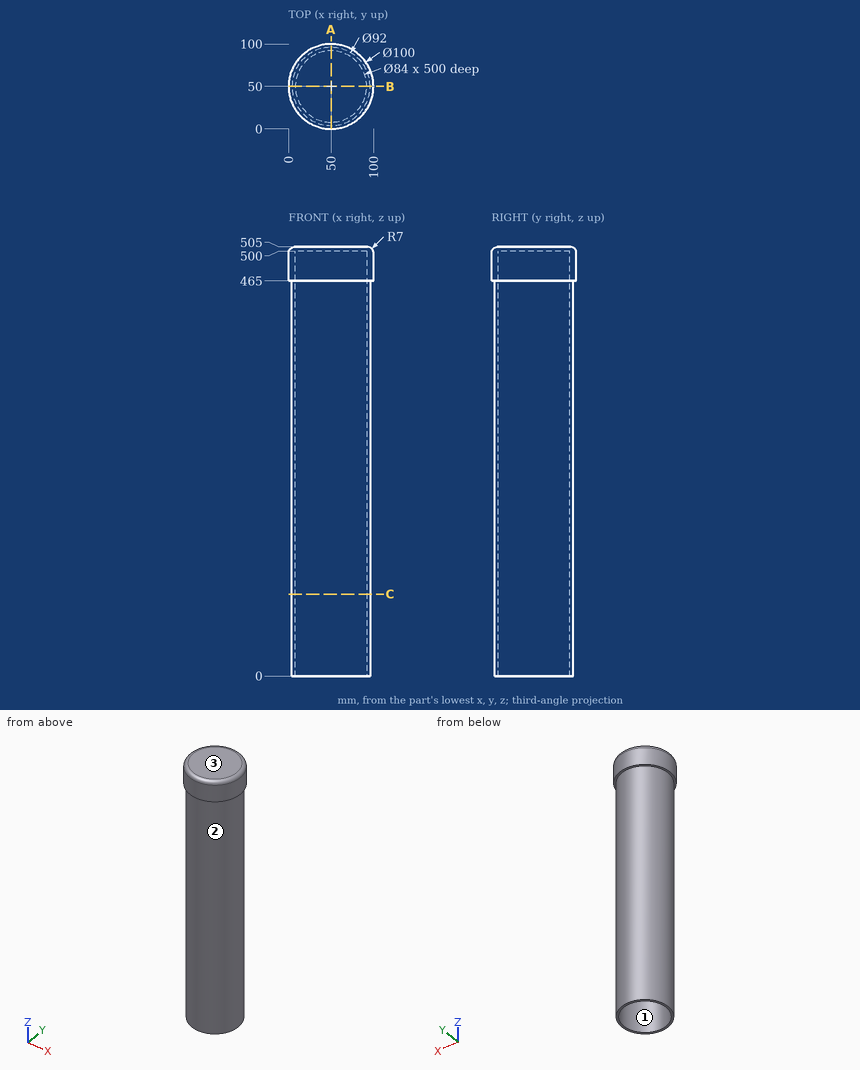
Design review of the part shown in the three views and the two pictorial views. Dimensions are in mm from the part's minimum x, y and z. Round coordinates to 2 decimals unless told otherwise and drop trailing zeros. Loops run counter-clockwise (first coordinate to the right, second up) from the corner with the lowest first, then second, coordinate; pieces in that order, holes last. Notation, with made-up numbers: (32.5, -26.75) - (37.5, -26.75) arc R27 cw to (37.5, -6.75) - close; hole circle Ø7 at (35.5, -34.5). An arc over 180 degrees is marked (long way). Write each question's results on one line, items separated by ' | '. Start each with the question number.
Q1. Take a section at C-C on z = 96.5. Give the boundary of the cut face in (x, y).
Q2. Wall thickness on line 1 along Y through (x, z) = (50, 174); line 2 along Y through (x, z) = (51, 470); line 3 along X through (y, z) = (26, 277): over which ranges is each line inside the solid? List them lowest first. Write a range as [from, to].
Q3. Take a section at A-A on x = 50. Give the boundary of the cut face in (y, z).
Q4. Draft analysis for pull direction Y (two halves, no side actions). For the marked faces 1, 2 and 3, state which applies: pulls with the +Y half, pulls with the -Y half, needs draft (parallel to the pull), parting line crosses it, or undercut.
Q5. Insertion check: P1, Ø25, axis at x = 36.5, y = 63.5, coming from the -Z side; P2, Ø3, axis at x = 43, z = 385, coming from the +Y side; P3, Ø1.5, axis at y = 18.5, z = 440, coming from the +X side. Each pin has a flat end and moves straight along its axis. Give the tip position at first contact, or say it passes through.
Data:
1) outline: circle Ø92 at (50, 50); hole circle Ø84 at (50, 50)
2) line 1: y = [4, 8], [92, 96] | line 2: y = [0.01, 8.01], [91.99, 99.99] | line 3: x = [10.76, 15.53], [84.47, 89.24]
3) outline: (0, 465) - (4, 465) - (4, 0) - (8, 0) - (8, 500) - (92, 500) - (92, 0) - (96, 0) - (96, 465) - (100, 465) - (100, 498) arc R7 ccw to (93, 505) - (7, 505) arc R7 ccw to (0, 498) - close
4) face 1: undercut | face 2: parting line crosses it | face 3: needs draft
5) P1: stops at z = 500 | P2: stops at y = 95.67 | P3: stops at x = 84.21
